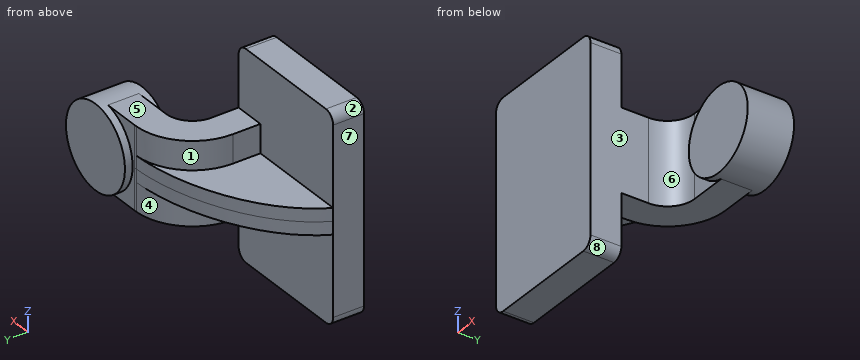
```python
from build123d import *

# Parameters (mm, degrees)
F1_DEPTH = 63.5
F0_W     = 25.0534382343
F0_H     = 19.05
F2_DEPTH = 25.4
F3_DEPTH = 7.9375
F5_R     = 6.35


with BuildPart() as f1:
    # F0 (on Top) → F1 (new body, symmetric)
    with BuildSketch(Plane.XY):
        Polygon((41.275, -9.525), (41.275, 9.525), (22.225, 9.525), (-41.275, 9.525), (-41.275, -9.525), align=None)
    extrude(amount=F1_DEPTH, both=True)

    # F0 (on Top) → F2 (join, symmetric)
    with BuildSketch(Plane.XY):
        with Locations((72.8517191172, 52.4002)):
            Rectangle(F0_W, F0_H)
        with BuildLine():
            Line((22.225, 9.525), (41.275, 9.525))
            Line((41.275, 9.525), (41.275, 26.3652))
            ThreePointArc((41.275, 26.3652), (46.1106670426, 38.0395329574), (57.785, 42.8752))
            Line((57.785, 42.8752), (60.325, 42.8752))
            Line((60.325, 42.8752), (60.325, 61.9252))
            Line((60.325, 61.9252), (57.785, 61.9252))
            add(Edge.make_bspline(
                [(56.4696013906, 61.9008627418), (56.9092910468, 61.9116915586), (57.3477786791, 61.9198078997), (57.785, 61.9252)],
                knots=[110.7361578147, 110.7361578147, 110.7361578147, 110.7361578147, 112.0654476636, 112.0654476636, 112.0654476636, 112.0654476636], degree=3))
            ThreePointArc((56.4696013906, 61.9008627418), (32.1794422581, 51.0404712797), (22.225, 26.3652))
            Line((22.225, 26.3652), (22.225, 9.525))
        make_face()
    extrude(amount=F2_DEPTH, both=True)

    # F0 (on Top) → F3 (join, symmetric)
    with BuildSketch(Plane.XY):
        with BuildLine():
            Line((-41.275, 9.525), (22.225, 9.525))
            Line((22.225, 9.525), (22.225, 26.3652))
            ThreePointArc((22.225, 26.3652), (32.1794422581, 51.0404712797), (56.4696013906, 61.9008627418))
            add(Edge.make_bspline(
                [(-41.275, 9.525), (-25.1285349977, 41.2729627023), (19.8413647419, 60.9987708748), (56.4696013906, 61.9008627418)],
                knots=[0, 0, 0, 0, 110.7361578147, 110.7361578147, 110.7361578147, 110.7361578147], degree=3))
        make_face()
    extrude(amount=F3_DEPTH, both=True)

    # F0 (on Top) → F4 (revolve)
    with BuildSketch(Plane.XY):
        Polygon((85.3784382343, 61.9252), (85.3784382343, 42.8752), (85.3784382343, 38.1), (111.125, 38.1), (111.125, 66.675), (85.3784382343, 66.675), align=None)
    revolve(axis=Axis((85.3784382343, 52.3875, 0), (0, -1, 0)))

    # F5
    f5_edges = [f1.edges().sort_by_distance(p)[0] for p in [
        (41.275, 0, 63.5),
        (-41.275, 0, 63.5),
        (41.275, 0, -63.5),
        (-41.275, 0, -63.5),
    ]]
    fillet(f5_edges, radius=F5_R)


solid = f1.part
```
Verification items for the finished model (mm, model axes). Face numbers are marked on the shaded views. A direction names the side the tool comes from. Give positions to 0.01 mm unless a question says otherwise; leave off trailing zeros. Loops run counter-clockwise (first coordinate to the right, second up) from the corner with the lowest first, then second, coordinate; pieces in that order, holes last.
1. Section check B-B, the plane z = 51. Enter the section's corners in (x, y) (3 decimals).
2. Section check A-A, the plane x = 63. Enter the section's corners in (y, z) (1 decimal).
3. Mould release check, pull along X, two halves, no side actions. Record for the marked faces 5, 6, 7 and 8: released by +X, released by -X, zero draft, split by the parting line, or undercut.
4. Go/stop test with flat-tipped pins: pin 1 Ø15.5 at (x, y) = (29, 26.5) entering from -Z; pin 2 Ø6 at (y, z) = (30.5, 3) entering from -X; pin 3 Ø5 at (y, z) = (15, -12.5) entering from -X (3 decimals). Record where each tip stops, or that it passes through.
5. Thickness scan on line 1 (Y direction, x = 81.5, z = 22) (3 decimals); line 2 (Y direction, x = 16, z = -57) (3 decimals); line 3 (X direction, y = 4, z = -47) (3 decimals). Record the ranges inside material, lowest first.
6. Set-up check for the marked faces 1, 2, 3 and 4: record each of +Z, -Z, +X, -X, +Y, -Y from which the full face is reachable in a straight line by a thin tool's end or side.
Geometry says:
1. outline: (-41.275, -9.525) - (41.275, -9.525) - (41.275, 9.525) - (-41.275, 9.525) - close
2. outline: (38.1, -12.7) - (42.9, -12.7) - (42.9, -25.4) - (61.9, -25.4) - (61.9, -12.7) - (66.7, -12.7) - (66.7, 12.7) - (61.9, 12.7) - (61.9, 25.4) - (42.9, 25.4) - (42.9, 12.7) - (38.1, 12.7) - close
3. face 5: zero draft
3. face 6: undercut
3. face 7: released by -X
3. face 8: released by +X
4. pin 1: stops at z = -25.4
4. pin 2: stops at x = -28.01
4. pin 3: stops at x = 22.225
5. line 1: y = 38.1 to 66.675
5. line 2: y = -9.525 to 9.525
5. line 3: x = -41.275 to 41.275
6. face 1: +Z, -X, +Y
6. face 2: +Z, -X, +Y, -Y
6. face 3: +Z, -Z, +X, -Y
6. face 4: -Z, -X, +Y
